Design review of the part built by this model. Coordinates are the model's own, in mm. Face numbers are marked on the shaded views. A direction names the side the tool comes from. Coordinates: 2 decimals unless noted, no trailing zeros. Loops run counter-clockwise (first coordinate to the right, second up) from the corner with the lowest first, then second, coordinate; pieces in that order, holes last. Notation, with made-up numbers: (84.5, 0.25) -> (107.5, 0.25) arc R17 ccw to (107.5, 12.25) -> close; hole circle Ø6 at (10, 35). An arc over 180 degrees is marked (long way). Answer as a JSON object with one key per item and string values.
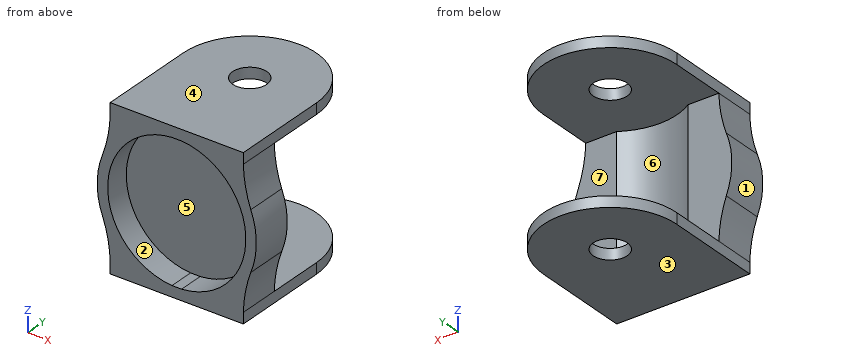
```python
from build123d import *

# Parameters (mm, degrees)
SKETCH1_R                  = 47.8
SKETCH1_R_2                = 41.5
CAP_BASE_DEPTH             = 15
SKETCH2_R                  = 47.8
CAP_TOP_DEPTH              = 10
SIDES_START                = 41.4
SIDES_DEPTH                = 6.5
SIDES_START_2              = -25
SIDES_TO_CAP_DEPTH         = 25
SKETCH5_R                  = 40.2
TRACKS_FOR_HOUSING_DEPTH   = 45
SKETCH6_R                  = 10.25
HOLE_FOR_GEAR_SHAFTS_DEPTH = 146.82002606


with BuildPart() as part:
    # Sketch1 → Cap base (new body)
    with BuildSketch(Plane(origin=(0, 0, 0), x_dir=(1, 0, 0), z_dir=(0, 1, 0))):
        with Locations(Location((0, 0, 0), (0, 0, 270))):
            Circle(SKETCH1_R)
        with Locations(Location((0, 0, 0), (0, 0, 270))):
            Circle(SKETCH1_R_2, mode=Mode.SUBTRACT)
    extrude(amount=CAP_BASE_DEPTH)

    # Sketch2 → Cap top (add)
    with BuildSketch(Plane(origin=(0, 15, 0), x_dir=(1, 0, 0), z_dir=(0, 1, 0))):
        with Locations(Location((0, 0, 0), (0, 0, 270))):
            Circle(SKETCH2_R)
    extrude(amount=CAP_TOP_DEPTH)

    # Sketch3 → Sides (add)
    with BuildSketch(Plane.XY.offset(SIDES_START)):
        with BuildLine():
            Line((-40, 59), (-40, 0))
            Line((-40, 0), (40, 0))
            Line((40, 0), (40, 59))
            ThreePointArc((40, 59), (0, 99), (-40, 59))
        make_face()
    sides = extrude(amount=SIDES_DEPTH)

    # Sketch4 → Sides to cap (add)
    with BuildSketch(Plane(origin=(0, 25, 0), x_dir=(1, 0, 0), z_dir=(0, 1, 0)).offset(SIDES_START_2)):
        with BuildLine():
            ThreePointArc((-23.893095237, -41.4), (-36.205132569, -31.209427673), (-44.469611721, -17.529792737))
            ThreePointArc((-44.469611721, -17.529792737), (-41.281194911, -29.286336098), (-40, -41.4))
            Line((-40, -41.4), (-23.893095237, -41.4))
        make_face()
        with BuildLine():
            Line((23.893095237, -41.4), (40, -41.4))
            ThreePointArc((40, -41.4), (41.281194911, -29.286336098), (44.469611721, -17.529792737))
            ThreePointArc((44.469611721, -17.529792737), (36.205132569, -31.209427673), (23.893095237, -41.4))
        make_face()
    sides_to_cap = extrude(amount=SIDES_TO_CAP_DEPTH)

    # Mirror1: Sides to cap across plane
    add(sides_to_cap.mirror(Plane.XY))

    # Mirror sides: Sides across plane
    add(sides.mirror(Plane.XY))

    # Sketch5 → Tracks for housing (cut)
    with BuildSketch(Plane(origin=(0, 0, 41.4), x_dir=(-1, 0, 0), z_dir=(0, 0, -1))):
        with Locations((0, 59)):
            Circle(SKETCH5_R)
    tracks_for_housing = extrude(amount=TRACKS_FOR_HOUSING_DEPTH, mode=Mode.SUBTRACT)

    # Mirror tracks: Tracks for housing across plane
    add(tracks_for_housing.mirror(Plane.XY), mode=Mode.SUBTRACT)

    # Sketch6 → Hole for gear shafts (cut, through all)
    with BuildSketch(Plane.XY.offset(47.9)):
        with Locations((0, 59)):
            Circle(SKETCH6_R)
    extrude(amount=-HOLE_FOR_GEAR_SHAFTS_DEPTH, mode=Mode.SUBTRACT)


solid = part.part
```
1) Add section B-B, the plane x = 0. Give the boundary of the cut face in (y, z), and give its area (3 significant figures).
Completed:
{"outline": "(0, -47.9) -> (48.75, -47.9) -> (48.75, -41.4) -> (18.8, -41.4) -> (18.8, 41.4) -> (48.75, 41.4) -> (48.75, 47.9) -> (0, 47.9) -> (0, 41.4) -> (15, 41.4) -> (15, -41.4) -> (0, -41.4) -> close; (69.25, -47.9) -> (99, -47.9) -> (99, -41.4) -> (69.25, -41.4) -> close; (69.25, 41.4) -> (99, 41.4) -> (99, 47.9) -> (69.25, 47.9) -> close", "area": "1,340 mm²"}
2) Add section C-C, the plane z = 0. Give the boundary of the cut face in (x, y), and give its area (3 significant figures).
Completed:
{"outline": "(-47.8, 0) -> (-41.5, 0) -> (-41.5, 15) -> (41.5, 15) -> (41.5, 0) -> (47.8, 0) -> (47.8, 25) -> (21.45, 25) arc R40.2 cw to (-21.45, 25) -> (-47.8, 25) -> close", "area": "965 mm²"}
3) Add section D-D, the plane x = 14.5. Give the boundary of the cut face in (y, z), and give its area (3 significant figures).
Completed:
{"outline": "(0, -47.9) -> (96.28, -47.9) -> (96.28, -41.4) -> (21.51, -41.4) -> (21.51, 41.4) -> (96.28, 41.4) -> (96.28, 47.9) -> (0, 47.9) -> (0, 38.88) -> (15, 38.88) -> (15, -38.88) -> (0, -38.88) -> close", "area": "1,870 mm²"}
4) The part is to be moulded in two halves that separate along X. For the marked faces 1, 2 and 3, say which applies: pulls with the +X half, pulls with the -X half, needs draft (parallel to the pull), parting line crosses it, or undercut.
Completed:
{"face 1": "pulls with the -X half", "face 2": "undercut", "face 3": "needs draft"}
5) Clearance check with flat-ended pins moving along their axes: pin 1 Ø3 at (y, z) = (32.5, -44.5) entering from -X; pin 2 Ø8 at (x, z) = (-32, 19) entering from +Y; pin 3 Ø2 at (y, z) = (28, -43) entering from +X; pin 4 Ø23.5 at (x, y) = (0, 59) entering from +Z. State where each tip first meets the part, or that it passes through.
Completed:
{"pin 1": "x = -40", "pin 2": "y = 25", "pin 3": "x = 40", "pin 4": "z = 47.9"}
6) Wall thickness on probe 1 along Y at (x, z) = (0, 44); probe 2 along Z at (x, y) = (4, 44.5); probe 3 along Y at (x, z) = (-35, 28): over which ranges is each line inside the solid? List them lowest first.
Completed:
{"probe 1": "0 to 48.75, 69.25 to 99", "probe 2": "-47.9 to -41.4, 41.4 to 47.9", "probe 3": "0 to 25"}
7) Add section A-A, the plane y = 28.5. Give the boundary of the cut face in (x, z).
Completed:
{"outline": "(-40, -47.9) -> (40, -47.9) -> (40, -41.4) -> (-40, -41.4) -> close; (-40, 41.4) -> (40, 41.4) -> (40, 47.9) -> (-40, 47.9) -> close"}
8) For the marked faces 4, 5, 6 and 7, list the 3-axis set-ups (+Z, -Z, +X, -X, +Y, -Y) from which the entire face can be reached by the end or side of a thin tool; tool diameter is ignored.
Completed:
{"face 4": "+Z, +X, -X, +Y, -Y", "face 5": "-Y", "face 6": "+Y", "face 7": "+X, -X, +Y"}
